For this review, take the finished solid that the model builds, in its own axes (mm). Face numbers are marked on the shaded views. A direction names the side the tool comes from. Give positions to 0.01 mm unless a question says otherwise; leave off trailing zeros. Write each loop counter-clockwise with the first axis right and the second up, starting at its lowest first coordinate (ties: lowest second). Pieces come first, ordered by that corner, then holes. Notation, with made-up numbers: (-19, 29.25) -> (17, 29.25) arc R31 ccw to (17, 56.25) -> close; hole circle Ø8 at (2, 12.25). An arc over 180 degrees is marked (long way). Return JSON: item names as keys, results as strings.
from build123d import *

# Parameters (mm, degrees)
SKETCH2_R             = 5
BOSS_EXTRUDE2_DEPTH   = 20
F_1_0MM_DOWEL_HOLE1_D = 10


with BuildPart() as part:
    # Sketch2 → Boss-Extrude2 (new body)
    with BuildSketch(Plane.XY):
        with BuildLine():
            Line((12.5, 131.912846307), (12.998411943, 163.796808069))
            ThreePointArc((12.998411943, 163.796808069), (0, 177), (-12.998411943, 163.796808069))
            Line((-12.998411943, 163.796808069), (-12.5, 131.912846307))
            ThreePointArc((-12.5, 131.912846307), (-13.474379896, 104.01025681), (-16.392772503, 76.243605923))
            Line((-16.392772503, 76.243605923), (-25, 15))
            Line((-25, 15), (-45, 15))
            Line((-45, 15), (-45, 0))
            Line((-45, 0), (-15, 0))
            ThreePointArc((-15, 0), (0, 15), (15, 0))
            Line((15, 0), (45, 0))
            Line((45, 0), (45, 15))
            Line((45, 15), (25, 15))
            Line((25, 15), (16.392772503, 76.243605923))
            ThreePointArc((16.392772503, 76.243605923), (13.474379896, 104.01025681), (12.5, 131.912846307))
        make_face()
        with Locations((0, 164)):
            Circle(SKETCH2_R, mode=Mode.SUBTRACT)
    extrude(amount=BOSS_EXTRUDE2_DEPTH)

    # Ø1.0mm Dowel Hole1 (through all)
    with Locations(Plane(origin=(0, 15, 0), x_dir=(1, 0, 0), z_dir=(0, 1, 0))):
        with Locations((-35, -10), (35, -10)):
            Hole(F_1_0MM_DOWEL_HOLE1_D / 2)


solid = part.part
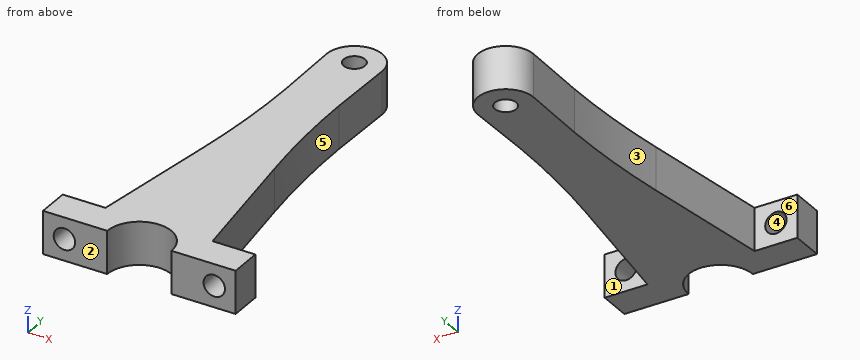
1. The part is to be moulded in two halves that separate along X. For the marked faces 4, 5 and 6, say which applies: +X half, -X half, draft (parallel to the pull), parting line (faces both ways), or undercut.
Results found:
{"face 4": "undercut", "face 5": "+X half", "face 6": "draft"}
2. Add section C-C, the plane x = 35. State the section outline as (y, z) points, plus the area to 3 significant figures.
Results found:
{"outline": "(0, 0) -> (15, 0) -> (15, 5) -> (0, 5) -> close; (0, 15) -> (15, 15) -> (15, 20) -> (0, 20) -> close", "area": "150 mm²"}
3. Add section B-B, the plane y = 13. State the section outline as (x, z) points.
Results found:
{"outline": "(-45, 0) -> (-7.48, 0) -> (-7.48, 20) -> (-45, 20) -> close; (7.48, 0) -> (45, 0) -> (45, 20) -> (7.48, 20) -> close; hole circle Ø10 at (-35, 10); hole circle Ø10 at (35, 10)"}
4. For the marked faces 1, 2 and 3, list the 3-axis set-ups (+Z, -Z, +X, -X, +Y, -Y) from which the entire face can be reached by the end or side of a thin tool; tool diameter is ignored.
Results found:
{"face 1": "+Z, -Z, +X, +Y", "face 2": "+Z, -Z, +X, -X, -Y", "face 3": "+Z, -Z, -X"}
5. For pin 1 (2 mm diameter, centred on y = 112.5, z = 18, fed in from -X); pin 2 (1 mm diameter, centred on x = 10.5, z = 2.5, fed in from +Y); pin 3 (2 mm diameter, centred on y = 18, z = 10, fed in from +X); pin 4 (3 mm diameter, centred on x = 35.5, z = 5, fed in from -Y), all flat-tipped, find the tip position at first contact; note any pin that passes through.
Results found:
{"pin 1": "stops at x = -13.02", "pin 2": "stops at y = 172.31", "pin 3": "stops at x = 24.72", "pin 4": "stops at y = 0"}
6. To check wall thickness, follow probe 1 along Z at (x, y) = (35, 8.5); probe 2 along X at (y, z) = (11.5, 10.75); probe 3 along Y at (x, z) = (0, 14.25). State the ranges of each line that lie inside material, in increasing order.
Results found:
{"probe 1": "z = 0 to 5, 15 to 20", "probe 2": "x = -45 to -39.94, -30.06 to -9.63, 9.63 to 30.06, 39.94 to 45", "probe 3": "y = 15 to 159, 169 to 177"}
7. Add section A-A, the plane z = 10. State the section outline as (x, y) points.
Results found:
{"outline": "(-45, 0) -> (-40, 0) -> (-40, 15) -> (-45, 15) -> close; (-30, 0) -> (-15, 0) arc R15 cw to (15, 0) -> (30, 0) -> (30, 15) -> (25, 15) -> (16.39, 76.24) arc R400 cw to (12.5, 131.91) -> (13, 163.8) arc R13 ccw (long way) to (-13, 163.8) -> (-12.5, 131.91) arc R400 cw to (-16.39, 76.24) -> (-25, 15) -> (-30, 15) -> close; (40, 0) -> (45, 0) -> (45, 15) -> (40, 15) -> close; hole circle Ø10 at (0, 164)"}
8. Add section D-D, the plane x = -0.5. State the section outline as (y, z) points.
Results found:
{"outline": "(14.99, 0) -> (159.03, 0) -> (159.03, 20) -> (14.99, 20) -> close; (168.97, 0) -> (176.99, 0) -> (176.99, 20) -> (168.97, 20) -> close"}
